```python
from build123d import *

# Parameters (mm, degrees)
F1_DEPTH = 50.8
F2_W     = 1.524
F2_H     = 5.08
F3_DEPTH = 50.8


with BuildPart() as f1:
    # F0 (on Top) → F1 (new body)
    with BuildSketch(Plane.XY):
        with BuildLine():
            Line((3.175, 0), (0, 0))
            Line((0, 0), (0, -74.295))
            ThreePointArc((0, -74.295), (2.417834, -80.132166), (8.255, -82.55))
            Line((8.255, -82.55), (10.795, -82.55))
            ThreePointArc((10.795, -82.55), (16.632166, -80.132166), (19.05, -74.295))
            Line((19.05, -74.295), (19.05, -66.675))
            Line((19.05, -66.675), (15.875, -66.675))
            Line((15.875, -66.675), (15.875, -74.295))
            ThreePointArc((15.875, -74.295), (14.387102, -77.887102), (10.795, -79.375))
            Line((10.795, -79.375), (8.255, -79.375))
            ThreePointArc((8.255, -79.375), (4.662898, -77.887102), (3.175, -74.295))
            Line((3.175, -74.295), (3.175, 0))
        make_face()
    extrude(amount=F1_DEPTH)

    # F2 (on face) → F3 (join)
    with BuildSketch(Plane(origin=(0, 0, 0), x_dir=(1, 0, 0), z_dir=(0, 0, -1))):
        with Locations((15.113, 69.215)):
            Rectangle(F2_W, F2_H)
    extrude(amount=-F3_DEPTH)


solid = f1.part
```
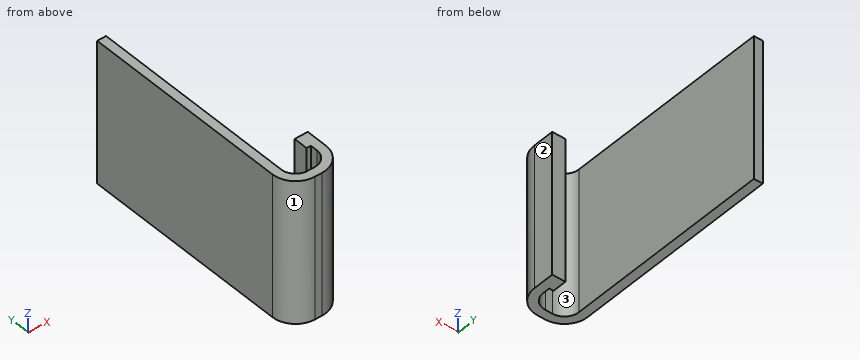
Input: part model. Units: mm. Frame: model coordinates. Face numbers are marked on the shaded views. Coordinates: 2 decimals unless noted, no trailing zeros. Loops run counter-clockwise (first coordinate to the right, second up) from the corner with the lowest first, then second, coordinate; pieces in that order, holes last. Notation, with made-up numbers: (18, 55) -> (52, 55) arc R22 ccw to (52, 89) -> close; hole circle Ø7 at (76, 82.5). An arc over 180 degrees is marked (long way). Use a Markdown table: item, result.
1) Material intervals for line 1 along X through (y, z) = (-62, 29) (3 decimals); line 2 along Y through (x, z) = (8.75, 41.5) (3 decimals); line 3 along Y through (x, z) = (11.25, 26), sorted ascending. Write a range as from..to.
Results found:
| item | result |
|---|---|
| line 1 | x = 0..3.175 |
| line 2 | y = -82.55..-79.375 |
| line 3 | y = -82.54..-79.35 |
2) Cut plane B-B (z = 47). Return the cut outline in (x, y) (3 decimals), then the cut area to 3 significant figures.
Results found:
| item | result |
|---|---|
| outline | (0, -74.295) arc R8.255 ccw to (8.255, -82.55) -> (10.795, -82.55) arc R8.255 ccw to (19.05, -74.295) -> (19.05, -66.675) -> (14.351, -66.675) -> (14.351, -71.755) -> (15.875, -71.755) -> (15.875, -74.295) arc R5.08 cw to (10.795, -79.375) -> (8.255, -79.375) arc R5.08 cw to (3.175, -74.295) -> (3.175, 0) -> (0, 0) -> close |
| area | 342 mm2 |
3) Cut plane A-A (y = -70). Return the cut outline in (x, z) (3 decimals).
Results found:
| item | result |
|---|---|
| outline | (0, 0) -> (3.175, 0) -> (3.175, 50.8) -> (0, 50.8) -> close; (14.351, 0) -> (19.05, 0) -> (19.05, 50.8) -> (14.351, 50.8) -> close |
4) Contact query for flat-ended pins moving along their axis: pin 1 (1.5 mm diameter, centred on x = 4, z = 36.5, fed in from -Y); pin 2 (4 mm diameter, centred on x = 14, z = 13, fed in from -Y); pin 3 (2 mm diameter, centred on x = 11, z = 6.5, fed in from +Y). Output: stop coordinate, or through.
Results found:
| item | result |
|---|---|
| pin 1 | stops at y = -81.77 |
| pin 2 | stops at y = -82.46 |
| pin 3 | stops at y = -79.23 |
5) Cut plane C-C (y = -58.5). Return the cut outline in (x, z) (3 decimals).
Results found:
| item | result |
|---|---|
| outline | (0, 0) -> (3.175, 0) -> (3.175, 50.8) -> (0, 50.8) -> close |
6) Pull-direction query (X, two-part tool) for the marked faces 1, 2 and 3; classes: released by +X, released by -X, zero draft, split by the parting line, or undercut.
Results found:
| item | result |
|---|---|
| face 1 | released by -X |
| face 2 | released by +X |
| face 3 | undercut |
7) Cut plane D-D (x = 9.5). Return the cut outline in (y, z) (3 decimals), then the cut area to 3 significant figures.
Results found:
| item | result |
|---|---|
| outline | (-82.55, 0) -> (-79.375, 0) -> (-79.375, 50.8) -> (-82.55, 50.8) -> close |
| area | 161 mm2 |
